Verification items for the finished model (mm, model axes). Face numbers are marked on the shaded views. A direction names the side the tool comes from. Round coordinates to 2 decimals unless told otherwise and drop trailing zeros. Loops run counter-clockwise (first coordinate to the right, second up) from the corner with the lowest first, then second, coordinate; pieces in that order, holes last. Notation, with made-up numbers: M 65,13.5 L 104,13.5 A19 cw 104,43.5 Z; hole C 27,42.25 d3. An arc over 180 degrees is marked long. Write item = value, one per line. Start each with the question number.
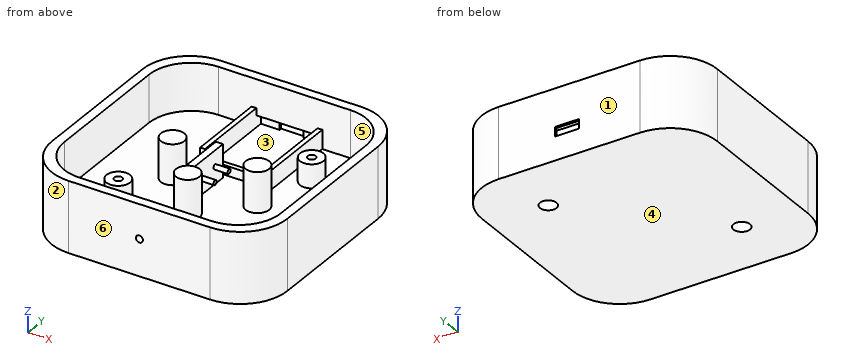
from build123d import *

# Parameters (mm, degrees)
CYLINDER009_R     = 1.5
CYLINDER009_DEPTH = 10
CYLINDER008_R     = 3.5
CYLINDER008_DEPTH = 8
CYLINDER006_R     = 1.7
CYLINDER006_DEPTH = 36
CYLINDER007_R     = 3.5
CYLINDER007_DEPTH = 8
CYLINDER005_R     = 1.7
CYLINDER005_DEPTH = 36
CYLINDER004_R     = 5
CYLINDER004_DEPTH = 10
CYLINDER003_R     = 5
CYLINDER003_DEPTH = 10
SKETCH002_W       = 19.8
SKETCH002_H       = 14
PAD001_DEPTH      = 3
SKETCH003_R       = 1
PAD002_DEPTH      = 6
CYLINDER_R        = 5
CYLINDER_DEPTH    = 17
CYLINDER001_R     = 5
CYLINDER001_DEPTH = 17
CYLINDER002_R     = 5
CYLINDER002_DEPTH = 17
BOX_W             = 2
BOX_H             = 34
BOX_DEPTH         = 10
BOX001_W          = 2
BOX001_H          = 34
BOX001_DEPTH      = 10
BOX004_W          = 30
BOX004_H          = 2
BOX004_DEPTH      = 6
BOX003_W          = 26
BOX003_H          = 10
BOX003_DEPTH      = 5
BOX002_W          = 10
BOX002_H          = 10
BOX002_DEPTH      = 4
PAD_DEPTH         = 30
POCKET_DEPTH      = 20


with BuildPart() as taladro_led:
    # Cylinder009 → Cylinder009 (new body)
    with BuildSketch(Plane(origin=(0, -44, 15.5), x_dir=(1, 0, 0), z_dir=(0, -1, 0))):
        Circle(CYLINDER009_R)
    extrude(amount=CYLINDER009_DEPTH)


with BuildPart() as cylinder008:
    # Cylinder008 → Cylinder008 (new body)
    with BuildSketch(Plane(origin=(25, 25, -4), x_dir=(1, 0, 0), z_dir=(0, 0, 1))):
        Circle(CYLINDER008_R)
    extrude(amount=CYLINDER008_DEPTH)


with BuildPart() as fusion002:
    # Cylinder006 → Cylinder006 (new body)
    with BuildSketch(Plane(origin=(25, 25, -4), x_dir=(1, 0, 0), z_dir=(0, 0, 1))):
        Circle(CYLINDER006_R)
    extrude(amount=CYLINDER006_DEPTH)

    # Fusion002: union Cylinder008
    add(cylinder008.part)


with BuildPart() as cylinder007:
    # Cylinder007 → Cylinder007 (new body)
    with BuildSketch(Plane(origin=(-25, -25, -4), x_dir=(1, 0, 0), z_dir=(0, 0, 1))):
        Circle(CYLINDER007_R)
    extrude(amount=CYLINDER007_DEPTH)


with BuildPart() as fusion001:
    # Cylinder005 → Cylinder005 (new body)
    with BuildSketch(Plane(origin=(-25, -25, -4), x_dir=(1, 0, 0), z_dir=(0, 0, 1))):
        Circle(CYLINDER005_R)
    extrude(amount=CYLINDER005_DEPTH)

    # Fusion001: union Cylinder007
    add(cylinder007.part)


with BuildPart() as cylinder004:
    # Cylinder004 → Cylinder004 (new body)
    with BuildSketch(Plane(origin=(25, 25, 10), x_dir=(1, 0, 0), z_dir=(0, 0, 1))):
        Circle(CYLINDER004_R)
    extrude(amount=CYLINDER004_DEPTH)


with BuildPart() as cylinder003:
    # Cylinder003 → Cylinder003 (new body)
    with BuildSketch(Plane(origin=(-25, -25, 10), x_dir=(1, 0, 0), z_dir=(0, 0, 1))):
        Circle(CYLINDER003_R)
    extrude(amount=CYLINDER003_DEPTH)


with BuildPart() as obj1:
    # Sketch002 → Pad001 (new body)
    with BuildSketch(Plane.YZ):
        with Locations((0, 7)):
            Rectangle(SKETCH002_W, SKETCH002_H)
    extrude(amount=PAD001_DEPTH)

    # Sketch003 (on Face6 of Pad001) → Pad002 (join)
    with BuildSketch(Plane.YZ.offset(3)):
        with Locations((-4.65, 7.2)):
            Circle(SKETCH003_R)
        with Locations((4.65, 7.2)):
            Circle(SKETCH003_R)
    extrude(amount=PAD002_DEPTH)


with BuildPart() as obj1_1:
    # Body002 placement: moved
    add(obj1.part.moved(Location((-6, 0, 10))))


with BuildPart() as cylinder:
    # Cylinder → Cylinder (new body)
    with BuildSketch(Plane(origin=(-18, 0, 10), x_dir=(1, 0, 0), z_dir=(0, 0, 1))):
        Circle(CYLINDER_R)
    extrude(amount=CYLINDER_DEPTH)


with BuildPart() as cylinder001:
    # Cylinder001 → Cylinder001 (new body)
    with BuildSketch(Plane(origin=(18, 0, 10), x_dir=(1, 0, 0), z_dir=(0, 0, 1))):
        Circle(CYLINDER001_R)
    extrude(amount=CYLINDER001_DEPTH)


with BuildPart() as cylinder002:
    # Cylinder002 → Cylinder002 (new body)
    with BuildSketch(Plane(origin=(0, -18, 10), x_dir=(1, 0, 0), z_dir=(0, 0, 1))):
        Circle(CYLINDER002_R)
    extrude(amount=CYLINDER002_DEPTH)


with BuildPart() as box:
    # Box → Box (new body)
    with BuildSketch(Plane(origin=(-14, 12, 8), x_dir=(1, 0, 0), z_dir=(0, 0, 1))):
        with Locations((1, 17)):
            Rectangle(BOX_W, BOX_H)
    extrude(amount=BOX_DEPTH)


with BuildPart() as box001:
    # Box001 → Box001 (new body)
    with BuildSketch(Plane(origin=(14, 12, 8), x_dir=(1, 0, 0), z_dir=(0, 0, 1))):
        with Locations((1, 17)):
            Rectangle(BOX001_W, BOX001_H)
    extrude(amount=BOX001_DEPTH)


with BuildPart() as box004:
    # Box004 → Box004 (new body)
    with BuildSketch(Plane(origin=(-14, 12, 8), x_dir=(1, 0, 0), z_dir=(0, 0, 1))):
        with Locations((15, 1)):
            Rectangle(BOX004_W, BOX004_H)
    extrude(amount=BOX004_DEPTH)


with BuildPart() as obj2:
    # Box003 → Box003 (new body)
    with BuildSketch(Plane(origin=(-12, 39, 10), x_dir=(1, 0, 0), z_dir=(0, 0, 1))):
        with Locations((13, 5)):
            Rectangle(BOX003_W, BOX003_H)
    extrude(amount=BOX003_DEPTH)


with BuildPart() as fusion:
    # Box002 → Box002 (new body)
    with BuildSketch(Plane(origin=(-4, 41, 10), x_dir=(1, 0, 0), z_dir=(0, 0, 1))):
        with Locations((5, 5)):
            Rectangle(BOX002_W, BOX002_H)
    extrude(amount=BOX002_DEPTH)

    # Fusion: union obj2
    add(obj2.part)


with BuildPart() as cut003:
    # Sketch → Pad (new body)
    with BuildSketch(Plane.XY):
        with BuildLine():
            Line((-30, 50), (30, 50))
            ThreePointArc((50, 30), (44.142136, 44.142136), (30, 50))
            Line((50, 30), (50, -30))
            ThreePointArc((30, -50), (44.142136, -44.142136), (50, -30))
            Line((30, -50), (-30, -50))
            ThreePointArc((-50, -30), (-44.142136, -44.142136), (-30, -50))
            Line((-50, -30), (-50, 30))
            ThreePointArc((-30, 50), (-44.142136, 44.142136), (-50, 30))
        make_face()
    extrude(amount=PAD_DEPTH)

    # Sketch001 (on Face10 of Pad) → Pocket (cut)
    with BuildSketch(Plane.XY.offset(30)):
        with BuildLine():
            Line((-28, 46), (28, 46))
            ThreePointArc((46, 28), (40.727922, 40.727922), (28, 46))
            Line((46, 28), (46, -28))
            ThreePointArc((28, -46), (40.727922, -40.727922), (46, -28))
            Line((28, -46), (-28, -46))
            ThreePointArc((-46, -28), (-40.727922, -40.727922), (-28, -46))
            Line((-46, -28), (-46, 28))
            ThreePointArc((-28, 46), (-40.727922, 40.727922), (-46, 28))
        make_face()
    extrude(amount=-POCKET_DEPTH, mode=Mode.SUBTRACT)

    # Cut: cut Fusion
    add(fusion.part, mode=Mode.SUBTRACT)

    # Fusion003: union Cylinder004, Cylinder003, obj1, Cylinder, Cylinder001, Cylinder002, Box, Box001, Box004
    add(cylinder004.part)
    add(cylinder003.part)
    add(obj1_1.part)
    add(cylinder.part)
    add(cylinder001.part)
    add(cylinder002.part)
    add(box.part)
    add(box001.part)
    add(box004.part)

    # Cut001: cut Fusion001
    add(fusion001.part, mode=Mode.SUBTRACT)

    # Cut002: cut Fusion002
    add(fusion002.part, mode=Mode.SUBTRACT)

    # Cut003: cut Taladro LED
    add(taladro_led.part, mode=Mode.SUBTRACT)


solid = cut003.part
1. Mould release check, pull along Y, two halves, no side actions. Record for the marked faces 1, 2, 3 and 4: pulls with the +Y half, pulls with the -Y half, needs draft (parallel to the pull), parting line crosses it, or undercut.
2. Section check C-C, the plane x = 25. Enter the section's corners in (y, z), and give its area (3 significant figures).
3. Tool access check on the marked faces 5 and 6. Record the directions out of +Z, -Z, +X, -X, +Y, -Y that give a thin tool (end or side, any length) a straight path to the whole face; none if there is none.
4. Thickness scan on line 1 (X direction, y = 14.5, z = 16); line 2 (Y direction, x = -25, z = 14.75); line 3 (X direction, y = 25, z = 1.95). Record the ranges inside material, lowest first.
5. Section check D-D, the plane x = -18. Enter the section's corners in (y, z).
6. Gauge pin test, flat ends, axial feed: P1, Ø3, axis at x = 24.5, y = 16.5, coming from the +Z side; P2, Ø3.5, axis at x = -24.5, y = -26, coming from the -Z side; P3, Ø10, axis at y = 37.5, z = 12, coming from the -X side. Record the tip position at first contact, or that the pin passes through.
7. Section check B-B, the plane y = -25. Enter the section's corners in (x, z).
8. Section check A-A, the plane z = 21.25. Enter the section's corners in (x, y), and give its area (3 significant figures).
Computed values:
q1.face_1 = pulls with the +Y half
q1.face_2 = pulls with the -Y half
q1.face_3 = undercut
q1.face_4 = needs draft
q2.outline = M -50,0 L 21.5,0 L 21.5,4 L 23.3,4 L 23.3,20 L 20,20 L 20,10 L -46,10 L -46,30 L -50,30 Z; M 26.7,4 L 28.5,4 L 28.5,0 L 50,0 L 50,30 L 46,30 L 46,10 L 30,10 L 30,20 L 26.7,20 Z
q2.area = 1,180 mm2
q3.face_5 = +Z
q3.face_6 = +Z, -Z, +X, -X, -Y
q4.line_1 = -50 to -46, -14 to -12, 14 to 16, 46 to 50
q4.line_2 = -50 to -46, -30 to -26.7, -23.3 to -20, 46 to 50
q4.line_3 = -50 to 21.5, 28.5 to 50
q5.outline = M -50,0 L 50,0 L 50,30 L 46,30 L 46,10 L 5,10 L 5,27 L -5,27 L -5,10 L -46,10 L -46,30 L -50,30 Z
q6.P1 = 10
q6.P2 = 4
q6.P3 = -49.84
q7.outline = M -50,0 L -28.5,0 L -28.5,4 L -26.7,4 L -26.7,20 L -30,20 L -30,10 L -46,10 L -46,30 L -50,30 Z; M -23.3,4 L -21.5,4 L -21.5,0 L 50,0 L 50,30 L 46,30 L 46,10 L -20,10 L -20,20 L -23.3,20 Z
q8.outline = M -50,-30 A20 ccw -30,-50 L 30,-50 A20 ccw 50,-30 L 50,30 A20 ccw 30,50 L -30,50 A20 ccw -50,30 Z; C -18,0 d10; M -6,-9.9 L -3,-9.9 L -3,9.9 L -6,9.9 Z; C 0,-18 d10; C 18,0 d10; hole M -46,-28 A18 ccw -28,-46 L 28,-46 A18 ccw 46,-28 L 46,28 A18 ccw 28,46 L -28,46 A18 ccw -46,28 Z
q8.area = 1,770 mm2
